Design review of the part built by this model. Coordinates are the model's own, in mm. Face numbers are marked on the shaded views. A direction names the side the tool comes from. Give positions to 0.01 mm unless a question says otherwise; leave off trailing zeros. Write each loop counter-clockwise with the first axis right and the second up, starting at its lowest first coordinate (ties: lowest second). Pieces come first, ordered by that corner, then holes. Notation, with made-up numbers: (-8.75, 8) -> (24.25, 8) arc R20 ccw to (24.25, 34) -> close; hole circle Ø6 at (51, -25). An arc over 180 degrees is marked (long way). Use CSV: the item, a comma, the result in double quotes.
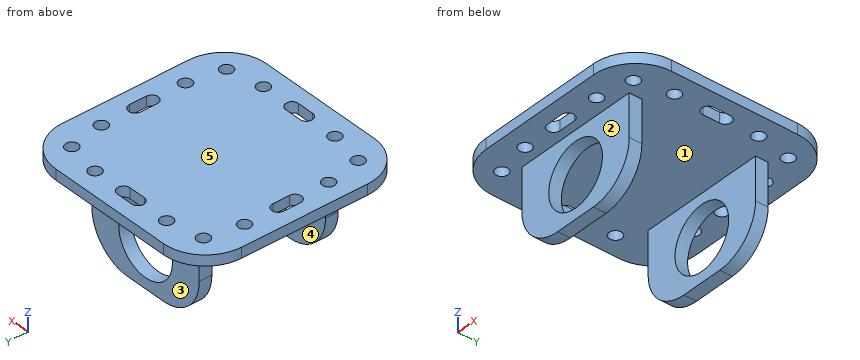
```python
from build123d import *

# Parameters (mm, degrees)
SKETCH1_W           = 50
SKETCH1_H           = 50
BOSS_EXTRUDE1_DEPTH = 2.5
SKETCH2_R           = 1.5
CUT_EXTRUDE1_DEPTH  = 5
FILLET1_R           = 10
SKETCH3_W           = 30
SKETCH3_H           = 3
BOSS_EXTRUDE2_DEPTH = 20
SKETCH4_R           = 7.5
CUT_EXTRUDE2_DEPTH  = 53.414215629
FILLET2_R           = 10


with BuildPart() as part:
    # Sketch1 → Boss-Extrude1 (new body)
    with BuildSketch(Plane.XY):
        Rectangle(SKETCH1_W, SKETCH1_H)
    extrude(amount=BOSS_EXTRUDE1_DEPTH)

    # Sketch2 → Cut-Extrude1 (cut)
    with BuildSketch(Plane(origin=(0, 0, 0), x_dir=(-1, 0, 0), z_dir=(0, 0, -1))):
        with Locations((18.384776311, 18.384776311)):
            Circle(SKETCH2_R)
        with Locations((18.384776311, -18.384776311)):
            Circle(SKETCH2_R)
        with Locations((-18.384776311, -18.384776311)):
            Circle(SKETCH2_R)
        with Locations((-18.384776311, 18.384776311)):
            Circle(SKETCH2_R)
        with Locations((20, 10)):
            Circle(SKETCH2_R)
        with Locations((20, -10)):
            Circle(SKETCH2_R)
        with Locations((-20, -10)):
            Circle(SKETCH2_R)
        with Locations((-20, 10)):
            Circle(SKETCH2_R)
        with Locations((10, 20)):
            Circle(SKETCH2_R)
        with Locations((-10, 20)):
            Circle(SKETCH2_R)
        with Locations((10, -20)):
            Circle(SKETCH2_R)
        with Locations((-10, -20)):
            Circle(SKETCH2_R)
        with BuildLine():
            Line((-2, 21.5), (2, 21.5))
            ThreePointArc((2, 21.5), (3.5, 20), (2, 18.5))
            Line((2, 18.5), (-2, 18.5))
            ThreePointArc((-2, 18.5), (-3.5, 20), (-2, 21.5))
        make_face()
        with BuildLine():
            Line((21.5, 2), (21.5, -2))
            ThreePointArc((21.5, -2), (20, -3.5), (18.5, -2))
            Line((18.5, -2), (18.5, 2))
            ThreePointArc((18.5, 2), (20, 3.5), (21.5, 2))
        make_face()
        with BuildLine():
            Line((2, -21.5), (-2, -21.5))
            ThreePointArc((-2, -21.5), (-3.5, -20), (-2, -18.5))
            Line((-2, -18.5), (2, -18.5))
            ThreePointArc((2, -18.5), (3.5, -20), (2, -21.5))
        make_face()
        with BuildLine():
            Line((-21.5, -2), (-21.5, 2))
            ThreePointArc((-21.5, 2), (-20, 3.5), (-18.5, 2))
            Line((-18.5, 2), (-18.5, -2))
            ThreePointArc((-18.5, -2), (-20, -3.5), (-21.5, -2))
        make_face()
    extrude(amount=-CUT_EXTRUDE1_DEPTH, mode=Mode.SUBTRACT)

    # Fillet1
    fillet1_edges = [part.edges().sort_by_distance(p)[0] for p in [
        (25, -25, 1.25),
        (-25, -25, 1.25),
        (-25, 25, 1.25),
        (25, 25, 1.25),
    ]]
    fillet(fillet1_edges, radius=FILLET1_R)

    # Sketch3 → Boss-Extrude2 (add)
    with BuildSketch(Plane(origin=(0, 0, 0), x_dir=(-1, 0, 0), z_dir=(0, 0, -1))):
        with Locations((0, 15)):
            Rectangle(SKETCH3_W, SKETCH3_H)
        with Locations((0, -15)):
            Rectangle(SKETCH3_W, SKETCH3_H)
    extrude(amount=BOSS_EXTRUDE2_DEPTH)

    # Sketch4 → Cut-Extrude2 (cut, through all)
    with BuildSketch(Plane.XZ.offset(16.5)):
        with Locations(Location((0, -10, 0), (0, 0, 270))):
            Circle(SKETCH4_R)
    extrude(amount=-CUT_EXTRUDE2_DEPTH, mode=Mode.SUBTRACT)

    # Fillet2
    fillet2_edges = [part.edges().sort_by_distance(p)[0] for p in [
        (-15, 15, -20),
        (15, 15, -20),
        (15, -15, -20),
        (-15, -15, -20),
    ]]
    fillet(fillet2_edges, radius=FILLET2_R)


solid = part.part
```
(1) Take a section at C-C (y = -10). Write out the cut boundary in (x, z).
Established:
outline,"(-25, 0) -> (-21.5, 0) -> (-21.5, 2.5) -> (-25, 2.5) -> close; (-18.5, 0) -> (18.5, 0) -> (18.5, 2.5) -> (-18.5, 2.5) -> close; (21.5, 0) -> (25, 0) -> (25, 2.5) -> (21.5, 2.5) -> close"
(2) Take a section at A-A (x = 0). Write out the cut boundary in (y, z).
Established:
outline,"(-25, 0) -> (-21.5, 0) -> (-21.5, 2.5) -> (-25, 2.5) -> close; (-18.5, 0) -> (-16.5, 0) -> (-16.5, -2.5) -> (-13.5, -2.5) -> (-13.5, 0) -> (13.5, 0) -> (13.5, -2.5) -> (16.5, -2.5) -> (16.5, 0) -> (18.5, 0) -> (18.5, 2.5) -> (-18.5, 2.5) -> close; (-16.5, -20) -> (-13.5, -20) -> (-13.5, -17.5) -> (-16.5, -17.5) -> close; (13.5, -20) -> (16.5, -20) -> (16.5, -17.5) -> (13.5, -17.5) -> close; (21.5, 0) -> (25, 0) -> (25, 2.5) -> (21.5, 2.5) -> close"
(3) For line 1 along Y through (x, z) = (10, 0.9); line 2 along Y through (x, z) = (-20, 1.35); line 3 along Y through (x, z) = (3.5, -18.5), list the stretches that pass through material, from the lowest coordinate up. Write a range as [from, to].
Established:
line 1,"y = [-25, -21.5], [-18.5, 18.5], [21.5, 25]"
line 2,"y = [-23.66, -11.5], [-8.5, -3.5], [3.5, 8.5], [11.5, 23.66]"
line 3,"y = [-16.5, -13.5], [13.5, 16.5]"
(4) Mouldability with a two-part tool opening along Y and no side actions: class the marked faces 1, 2 and 3 as +Y half, -Y half, draft (parallel to the pull), parting line (faces both ways), or undercut.
Established:
face 1,"undercut"
face 2,"-Y half"
face 3,"+Y half"
(5) Clearance check with flat-ended pins moving along their axes: pin 1 (1.5 mm diameter, centred on y = -15.5, z = -4.5, fed in from -X); pin 2 (1.5 mm diameter, centred on x = -11.5, z = -7, fed in from -Y); pin 3 (2 mm diameter, centred on x = 8.5, y = -4.5, fed in from -Z); pin 4 (13.5 mm diameter, centred on x = 0, z = -10, fed in from -Y). State where each tip first meets the part, or that it passes through.
Established:
pin 1,"stops at x = -15"
pin 2,"stops at y = -16.5"
pin 3,"stops at z = 0"
pin 4,"passes through"
(6) Take a section at D-D (x = -10). Write out the cut boundary in (y, z).
Established:
outline,"(-25, 0) -> (-21.5, 0) -> (-21.5, 2.5) -> (-25, 2.5) -> close; (-18.5, 0) -> (-16.5, 0) -> (-16.5, -18.66) -> (-13.5, -18.66) -> (-13.5, 0) -> (13.5, 0) -> (13.5, -18.66) -> (16.5, -18.66) -> (16.5, 0) -> (18.5, 0) -> (18.5, 2.5) -> (-18.5, 2.5) -> close; (21.5, 0) -> (25, 0) -> (25, 2.5) -> (21.5, 2.5) -> close"
(7) Take a section at B-B (z = -4). Write out the cut boundary in (x, y).
Established:
outline,"(-15, -16.5) -> (-4.5, -16.5) -> (-4.5, -13.5) -> (-15, -13.5) -> close; (-15, 13.5) -> (-4.5, 13.5) -> (-4.5, 16.5) -> (-15, 16.5) -> close; (4.5, -16.5) -> (15, -16.5) -> (15, -13.5) -> (4.5, -13.5) -> close; (4.5, 13.5) -> (15, 13.5) -> (15, 16.5) -> (4.5, 16.5) -> close"
(8) Tool access review of the marked faces 4 and 5: name each direction out of +Z, -Z, +X, -X, +Y, -Y from which nothing blocks a thin tool from reaching the whole face with its end or side.
Established:
face 4,"-Z, +X, -X"
face 5,"+Z, +X, -X, +Y, -Y"
